Input: part model. Units: mm. Frame: model coordinates. A direction names the side the tool comes from. Round coordinates to 2 decimals unless told otherwise and drop trailing zeros. Order: outer loops, then holes, each group sorted by start corner. A loop starts at its lowest first (then second) coordinate and runs counter-clockwise, first axis right, second up. Notation, with made-up numbers: (61, -0.75) -> (74, -0.75) arc R14 ccw to (74, 14.25) -> close; hole circle Ø11 at (34, -40). An arc over 180 degrees is marked (long way). Answer as CSV lines item,"result". Start each with the question number.
1) Section query A-A, the plane z = 31.5. Output: boundary loops of the cut face in (x, y), and give its area (3 significant figures).
2) Section query C-C, the plane x = 44.5. Output: boundary loops of the cut face in (y, z).
3) Mould query, pull axis X, two halves, no side actions, for faces 1 (the face through (-1.5, 0, -22)), 2 (the face through (-12, 0, 1.5)), 3 (the face through (47.497, 20.77, -0.021)). Classes: +X half, -X half, draft (parallel to the pull), parting line (faces both ways), or undercut.
4) Section query D-D, the plane y = -14. Output: boundary loops of the cut face in (x, z).
5) Line query: L1, parallel to X at y = -22, z = -32; L2, parallel to Y at x = 44.5, z = 0.35; L3, parallel to Z at x = 0.4, y = -20. Output: solid intervals per line, ascending.
6) Section query B-B, the plane z = -16. Output: boundary loops of the cut face in (x, y).
7) Access query for faces 4 (the face through (34, 0, -1.5)), 5 (the face through (11.5, 0, -21)), 6 (the face through (-12, 0, -1.5)). Directions: +Z, -Z, +X, -X, +Y, -Y. A direction counts if a zero-diameter tool reaches every point of the face in a straight line with its end or side. Return the directions, or none.
8) First-contact query: P1, Ø6, axis at x = -13, y = -14.5, coming from the -Z side; P2, Ø7, axis at x = 44.5, y = 20.64, coming from the +Z side; P3, Ø3.5, axis at x = 44.5, y = -20.64, coming from the +Z side; P4, Ø12, axis at y = 12.5, z = -21.5, coming from the +X side. Flat tips, straight axial feed; report the tip coordinate or a pass-through.
```python
from build123d import *

# Parameters (mm, degrees)
F0_W          = 3
F0_H          = 40
F0_H_2        = 3
F0_W_2        = 20
F0_W_3        = 10
F0_W_4        = 7
F0_W_5        = 33
F1_DEPTH      = 30
F1_DEPTH_BACK = 30
F3_D          = 6
F3_DEPTH      = 12
F3_TIP        = 1.8025818571
F5_D          = 6
F5_DEPTH      = 12
F5_TIP        = 1.8025818571


with BuildPart() as f1:
    # F0 (on Front) → F1 (new body, two sides)
    with BuildSketch(Plane.XZ) as f1_sk:
        with Locations((0, 21.5)):
            Rectangle(F0_W, F0_H)
        Rectangle(F0_W, F0_H_2)
        with Locations((-11.5, 0)):
            Rectangle(F0_W_2, F0_H_2)
        with Locations((6.5, 0)):
            Rectangle(F0_W_3, F0_H_2)
        with Locations((0, -21.5)):
            Rectangle(F0_W, F0_H)
        with Locations((13, 0)):
            Rectangle(F0_W, F0_H_2)
        Polygon((14.5, -1.5), (11.5, -1.5), (11.5, -8.7749995426), (11.5, -41.5), (14.5, -41.5), (14.5, -8.7749995426), align=None)
        with Locations((18, 0)):
            Rectangle(F0_W_4, F0_H_2)
        with Locations((38, 0)):
            Rectangle(F0_W_5, F0_H_2)
    extrude(amount=F1_DEPTH)
    extrude(f1_sk.sketch, amount=-F1_DEPTH_BACK)

    # F3
    with Locations(Plane.YZ.offset(1.5)):
        with Locations((-20, 31.5), (20, 31.5)):
            Hole(F3_D / 2, depth=F3_DEPTH)
            with Locations((0, 0, -(F3_DEPTH + F3_TIP / 2))):  # 118° drill point
                Cone(0, F3_D / 2, F3_TIP, mode=Mode.SUBTRACT)

    # F5
    with Locations(Plane.XY.offset(1.5)):
        with Locations((44.5, 20.6381995231), (44.5, -20.6381995231)):
            Hole(F5_D / 2, depth=F5_DEPTH)
            with Locations((0, 0, -(F5_DEPTH + F5_TIP / 2))):  # 118° drill point
                Cone(0, F5_D / 2, F5_TIP, mode=Mode.SUBTRACT)


solid = f1.part
```
Findings:
1,outline,"(-1.5, -30) -> (1.5, -30) -> (1.5, -23) -> (-1.5, -23) -> close; (-1.5, -17) -> (1.5, -17) -> (1.5, 17) -> (-1.5, 17) -> close; (-1.5, 23) -> (1.5, 23) -> (1.5, 30) -> (-1.5, 30) -> close"
1,area,"144 mm^2"
2,outline,"(-30, -1.5) -> (-23.64, -1.5) -> (-23.64, 1.5) -> (-30, 1.5) -> close; (-17.64, -1.5) -> (17.64, -1.5) -> (17.64, 1.5) -> (-17.64, 1.5) -> close; (23.64, -1.5) -> (30, -1.5) -> (30, 1.5) -> (23.64, 1.5) -> close"
3,face 1,"-X half"
3,face 2,"draft"
3,face 3,"undercut"
4,outline,"(-21.5, -1.5) -> (-1.5, -1.5) -> (-1.5, -41.5) -> (1.5, -41.5) -> (1.5, -1.5) -> (11.5, -1.5) -> (11.5, -41.5) -> (14.5, -41.5) -> (14.5, -1.5) -> (54.5, -1.5) -> (54.5, 1.5) -> (1.5, 1.5) -> (1.5, 41.5) -> (-1.5, 41.5) -> (-1.5, 1.5) -> (-21.5, 1.5) -> close"
5,L1,"x = -1.5 to 1.5, 11.5 to 14.5"
5,L2,"y = -30 to -23.64, -17.64 to 17.64, 23.64 to 30"
5,L3,"z = -41.5 to 28.5, 34.5 to 41.5"
6,outline,"(-1.5, -30) -> (1.5, -30) -> (1.5, 30) -> (-1.5, 30) -> close; (11.5, -30) -> (14.5, -30) -> (14.5, 30) -> (11.5, 30) -> close"
7,face 4,"-Z, +X, +Y, -Y"
7,face 5,"-Z, +Y, -Y"
7,face 6,"-Z, -X, +Y, -Y"
8,P1,"stops at z = -1.5"
8,P2,"stops at z = 1.5"
8,P3,"passes through"
8,P4,"stops at x = 14.5"
